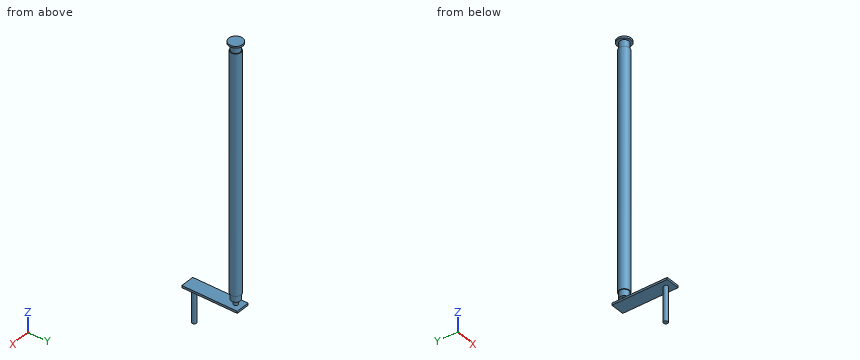
Autodesk Inventor part; units mm, degrees
ref_plane "YZ Plane" through (0, 0, 0) normal (1, 0, 0) x (0, 1, 0)
ref_plane "XZ Plane" through (0, 0, 0) normal (0, 1, 0) x (-1, 0, 0)
ref_plane "XY Plane" through (0, 0, 0) normal (0, 0, 1) x (1, 0, 0)
sketch "Sketch1" plane through (0, 0, 0) normal (0, 0, 1) x (1, 0, 0)
  circle A0 centre (0, 0) radius 25
  dimension "d0" = 50
extrude "Extrusion1" add sketch "Sketch1" along normal blind 10
sketch "Sketch2" plane through (0, 0, 10) normal (0, 0, 1) x (1, 0, 0)
  circle A0 centre (0, 0) radius 6.5
  dimension "d3" = 13
extrude "Extrusion2" add sketch "Sketch2" along normal blind 10
fillet "Fillet1" radius 1 1 edges at (-6.5, 0, 10)
sketch "Sketch4" plane through (0, 0, 0) normal (0, 0, -1) x (-1, 0, 0)
  arc A0 (19.3649, 5) -> (5, 19.3649) centre (0, 0) ccw
  line L0 (2.5, 17.4284) -> (2.5, 9.4868)
  line L1 (9.4868, 2.5) -> (17.4284, 2.5)
  arc A1 (5, 19.3649) -> (2.5, 17.4284) centre (4.5, 17.4284) ccw
  arc A2 (17.4284, 2.5) -> (19.3649, 5) centre (17.4284, 4.5) ccw
  arc A3 (2.5, 8.3666) -> (2.5153, 8.1193) centre (4.5, 8.3666) ccw
  arc A4 (8.1193, 2.5153) -> (8.3666, 2.5) centre (8.3666, 4.5) ccw
  arc A5 (7.6798, 3.6429) -> (3.6429, 7.6798) centre (0, 0) ccw
  arc A6 (2.5, 9.4868) -> (3.6429, 7.6798) centre (4.5, 9.4868) ccw
  arc A7 (7.6798, 3.6429) -> (9.4868, 2.5) centre (9.4868, 4.5) ccw
  point P0 (2.5, 19.8431)
  point P1 (19.8431, 2.5)
  point P2 (2.5, 7.0711)
  point P3 (7.0711, 2.5)
extrude "Extrusion3" cut sketch "Sketch4" against normal blind 10
pattern_circular "Circular Pattern1" count 4 over 360 about axis through (0, 0, 11) along (0, 0, -1) of "Extrusion3"
sketch "Sketch7" plane through (0, 0, 20) normal (0, 0, 1) x (1, 0, 0)
  circle A0 centre (0, 0) radius 7.5
  dimension "d38" = 15
extrude "Extrusion5" add sketch "Sketch7" along normal blind 340
sketch "Sketch8" plane through (0, 0, 360) normal (0, 0, 1) x (1, 0, 0)
  circle A0 centre (0, 0) radius 6.5
  dimension "d41" = 13
extrude "Extrusion6" add sketch "Sketch8" along normal blind 10
sketch "Sketch9" plane through (0, 0, 370) normal (0, 0, 1) x (1, 0, 0)
  circle A0 centre (0, 0) radius 10
  dimension "d44" = 20
extrude "Extrusion7" add sketch "Sketch9" along normal blind 2.5
thread "Thread1"
sketch "Sketch10" plane through (0, 0, 0) normal (0, 0, -1) x (-1, 0, 0)
  circle A0 centre (0, 0) radius 25
extrude "Extrusion8" cut sketch "Sketch10" against normal blind 11
sketch "Sketch11" plane through (0, 0, 11) normal (0, 0, -1) x (-1, 0, 0)
  circle A0 centre (0, 0) radius 3
  dimension "d51" = 6
extrude "Extrusion9" add sketch "Sketch11" along normal blind 10
sketch "Sketch12" plane through (0, 0, 1) normal (0, 0, -1) x (-1, 0, 0)
  circle A0 centre (0, 0) radius 3
  circle A1 centre (0, 0) radius 3
  line L0 (-10, 10) -> (10, 10)
  line L1 (10, 10) -> (10, -70)
  line L2 (10, -70) -> (-10, -70)
  line L3 (-10, -70) -> (-10, 10)
  dimension "d54" = 20
  dimension "d55" = 80
extrude "Extrusion10" add sketch "Sketch12" against normal blind 3
sketch "Sketch13" plane through (0, 0, 1) normal (0, 0, -1) x (-1, 0, 0)
  line L0 (10, -70) -> (-10, -70)
  circle A0 centre (0, -60) radius 3
  point P0 (0, 0)
  dimension "d59" = 6
extrude "Extrusion11" add sketch "Sketch13" along normal blind 50
properties part number "leadscrew_modified" material "Steel, Alloy"
Verification items for the finished model (mm, model axes). Coordinates: 2 decimals unless noted, no trailing zeros. Order: outer loops, then holes, each group sorted by start corner. A loop starts at its lowest first (then second) coordinate and runs counter-clockwise, first axis right, second up. Notation, with made-up numbers: (-37, 13.25) -> (-19, 13.25) arc R35 cw to (-19, 47.25) -> close; hole circle Ø10 at (5, -15.5). An arc over 180 degrees is marked (long way). Use CSV: the item, a comma, the result in double quotes. Start each with the question number.
Q1. Section check C-C, the plane y = -19. Record the cut outline in (x, z).
Q2. Thickness scan on line 1 along Z through (x, y) = (-1.75, -60.5); line 2 along Y through (x, z) = (-0.5, 43); line 3 along Z through (x, y) = (0.75, -25.5). Record the ranges inside material, lowest first.
Q3. Section check A-A, the plane x = 0. Record the cut outline in (y, z).
Q4. Section check B-B, the plane z = 224.5. Record the cut outline in (x, y).
Q5. Depth check by flat-ended pin: P1, Ø1.5, axis at x = 5, y = -11, coming from the +Z side; P2, Ø10, axis at y = -10.5, z = 237.5, coming from the -X side; P3, Ø10, axis at x = -4, z = 54, coming from the +Y side. Enter the tip coordinate at first touch or a pass-through.
Returned:
1,outline,"(-10, 1) -> (10, 1) -> (10, 4) -> (-10, 4) -> close"
2,line 1,"z = -49 to 4"
2,line 2,"y = -7.48 to 7.48"
2,line 3,"z = 1 to 4"
3,outline,"(-70, 1) -> (-63, 1) -> (-63, -49) -> (-57, -49) -> (-57, 1) -> (10, 1) -> (10, 4) -> (3, 4) -> (3, 11) -> (6.5, 11) -> (6.5, 20) -> (7.5, 20) -> (7.5, 360) -> (6.5, 360) -> (6.5, 370) -> (10, 370) -> (10, 372.5) -> (-10, 372.5) -> (-10, 370) -> (-6.5, 370) -> (-6.5, 360) -> (-7.5, 360) -> (-7.5, 20) -> (-6.5, 20) -> (-6.5, 11) -> (-3, 11) -> (-3, 4) -> (-70, 4) -> close"
4,outline,"circle Ø15 at (0, 0)"
5,P1,"stops at z = 4"
5,P2,"stops at x = -5.1"
5,P3,"stops at y = 7.5"
